Could you check a few things on this model? Use its own coordinates, in mm. A direction names the side the tool comes from. Give positions to 0.01 mm unless a question says otherwise; leave off trailing zeros. Answer in a Markdown table with one row per item. Add a question column.
1. Thinking about a two-plate mould opening in Y: for faces 1 (the flat face through (-1.18, 17.01, 6.1)), 2 (the cylindrical face through (-1.359, -16.199, -9.938)), 3 (the flat face through (-1.18, 14.94, -10.18)), which applies, released by +Y, released by -Y, zero draft, split by the parting line, or undercut?
2. I'm going to push flat-ended pins straight in: pin 1 Ø6 at (x, z) = (-2.5, 9.5) entering from +Y; pin 2 Ø16.5 at (y, z) = (0, 0) entering from -X; pin 3 Ø2 at (x, z) = (-4, 3) entering from -Y. Where does each tip first touch, or does it pass through?
3. Which directions (+Z, -Z, +X, -X, +Y, -Y) give clear straight access to the entire face, cutting with the end or side of a thin tool? Please do faces 4 (the flat face through (-1.18, 8.67, 15.83)), 5 (the flat face through (-1.181, -3.353, -17.735)), 6 (the flat face through (-1.181, 17.735, -3.353)).
4. I need wall thicknesses on line 1 along Y through (x, z) = (-1.15, 0); line 2 along Y through (x, z) = (-6.5, 0). Which ranges of each line are inside material? Lowest first, please. Write a range as from..to.
```python
from build123d import *

# Parameters (mm, degrees)
F3_DEPTH = 25.4
F4_COUNT = 40


with BuildPart() as f1:
    # F0 (on Top) → F1 (revolve)
    with BuildSketch(Plane.XY):
        Polygon((-2.54, 15.24), (0, 15.24), (3.2612350769, 15.24), (5.08, 15.24), (5.08, 19.0043579787), (-7.62, 19.0043579787), (-7.62, 15.24), (-5.8012350769, 15.24), align=None)
        with BuildLine():
            ThreePointArc((-5.8012350769, 15.24), (-3.4715579779, 14.0044093291), (-2.54, 11.5373707349))
            Line((-2.54, 11.5373707349), (-2.54, 15.24))
            Line((-2.54, 15.24), (-5.8012350769, 15.24))
        make_face()
        Polygon((-2.54, 5.08), (0, 5.08), (0, 11.5373707349), (0, 15.24), (-2.54, 15.24), (-2.54, 11.5373707349), align=None)
        with BuildLine():
            Line((0, 15.24), (0, 11.5373707349))
            ThreePointArc((0, 11.5373707349), (0.9315579779, 14.0044093291), (3.2612350769, 15.24))
            Line((3.2612350769, 15.24), (0, 15.24))
        make_face()
    revolve(axis=Axis((-6.35, 0, 0), (-1, 0, 0)))

    # F2 (on face) → F3 (cut)
    with BuildSketch(Plane.YZ.offset(5.08)):
        with BuildLine():
            Line((0, 17.1221789894), (0, 19.0043579787))
            ThreePointArc((0, 19.0043579787), (-0.4103514296, 18.9999272074), (-0.8205115163, 18.9866369596))
            Line((-0.8205115163, 18.9866369596), (-0.2629475493, 17.1221789894))
            Line((-0.2629475493, 17.1221789894), (0, 17.1221789894))
        make_face()
        with BuildLine():
            ThreePointArc((0.8205115163, 18.9866369596), (0.4103514296, 18.9999272074), (0, 19.0043579787))
            Line((0, 19.0043579787), (0, 17.1221789894))
            Line((0, 17.1221789894), (0.2629475493, 17.1221789894))
            Line((0.2629475493, 17.1221789894), (0.8205115163, 18.9866369596))
        make_face()
    f3 = extrude(amount=-F3_DEPTH, mode=Mode.SUBTRACT)

    # F4: F3 ×40 about axis
    f4_axis = Axis((0, 0, 0), (-1, 0, 0))
    for i in range(1, F4_COUNT):
        add(f3.rotate(f4_axis, i * 360 / F4_COUNT), mode=Mode.SUBTRACT)


solid = f1.part
```
Results:
| question | item | result |
|---|---|---|
| 1 | face 1 | released by +Y |
| 1 | face 2 | released by -Y |
| 1 | face 3 | undercut |
| 2 | pin 1 | y = 17.8 |
| 2 | pin 2 | x = -2.54 |
| 2 | pin 3 | y = -18.9 |
| 3 | face 4 | +Z, +X, -X |
| 3 | face 5 | -Z, +X, -X |
| 3 | face 6 | +X, -X, +Y |
| 4 | line 1 | -17.12..-5.08, 5.08..17.12 |
| 4 | line 2 | -17.12..-15.24, 15.24..17.12 |
